Verification items for the finished model (mm, model axes). A direction names the side the tool comes from. Give positions to 0.01 mm unless a question says otherwise; leave off trailing zeros. Write each loop counter-clockwise with the first axis right and the second up, starting at its lowest first coordinate (ties: lowest second). Pieces come first, ordered by that corner, then holes.
Autodesk Inventor part; units mm, degrees
ref_plane "YZ Plane" through (0, 0, 0) normal (1, 0, 0) x (0, 1, 0)
ref_plane "XZ Plane" through (0, 0, 0) normal (0, 1, 0) x (-1, 0, 0)
ref_plane "XY Plane" through (0, 0, 0) normal (0, 0, 1) x (1, 0, 0)
sketch "Sketch1" plane through (0, 0, 0) normal (0, 0, 1) x (1, 0, 0)
  circle A0 centre (0, 0) radius 30.099
  dimension "d0" = 60.198
extrude "Extrusion1" add sketch "Sketch1" along normal blind 6.1468
sketch "Sketch2" plane through (0, 0, 0) normal (0, 0, -1) x (-1, 0, 0)
  circle A0 centre (0, 0) radius 21.3106
  dimension "d3" = 42.6212
extrude "Extrusion2" add sketch "Sketch2" along normal blind 5.08
sketch "Sketch3" plane through (0, 0, 0) normal (0, 0, -1) x (-1, 0, 0)
  circle A0 centre (0, 0) radius 21.3106
  circle A1 centre (0, 0) radius 30.099
  line L0 (0, 25.4139) -> (22.0091, -12.707) construction
  line L1 (22.0091, -12.707) -> (-22.0091, -12.707) construction
  line L2 (-22.0091, -12.707) -> (0, 25.4139) construction
  circle A2 centre (0, 25.4139) radius 1.4224
  circle A3 centre (22.0091, -12.707) radius 1.4224
  circle A4 centre (-22.0091, -12.707) radius 1.4224
  line L3 (-11.071, 20.6645) -> (5.4814, 30.221) construction
  line L4 (36.2551, -6.1245) -> (10.9127, -20.7559) construction
  dimension "d6" = 44.0182
  dimension "d7" = 2.8448
  dimension "d8" = 46.863
extrude "Extrusion3" add sketch "Sketch3" along normal blind 8.6868 contours A2 | A3 | A4
sketch "Sketch4" plane through (0, 0, 0) normal (1, 0, 0) x (0, 1, 0)
  line L0 (30.099, 6.1468) -> (-30.099, 6.1468)
  line L1 (27.2941, 6.1468) -> (19.2856, 15.3189)
  line L2 (19.2856, 15.3189) -> (19.2856, 28.4756)
  line L3 (19.2856, 28.4756) -> (0, 28.4756)
  line L4 (0, 28.4756) -> (0, 0)
  point P0 (0, 6.1468)
revolve "Revolution1" add sketch "Sketch4" angle 360 about axis through (0, 0, 28.4756) along (0, 0, -1)
sketch "Sketch5" plane through (0, 0, 28.4756) normal (0, 0, 1) x (1, 0, 0)
  circle A0 centre (0, -14.4677) radius 2.7154
  point P0 (0, 0)
extrude "Extrusion4" add sketch "Sketch5" along normal blind 16.6243
properties part number "MPG"
Item 1: Depth check by flat-ended pin: pin 1 (6 mm diameter, centred on x = 21.5, y = 19.5, fed in from -Z); pin 2 (12 mm diameter, centred on x = -3, y = -5, fed in from -Z); pin 3 (12 mm diameter, centred on y = -15, z = 13, fed in from +X). Enter the tip coordinate at first touch or a pass-through.
Answer key:
pin 1: stops at z = 0
pin 2: stops at z = -5.08
pin 3: stops at x = 22.9
Item 2: Release check for a two-part mould opening along Y. For faces 1 (the face through (-0.656, 26.676, -4.283)), 2 (the face through (0, 0, -5.08)), 3 (the face through (18.827, -4.181, 21.989)) record: released by +Y, released by -Y, zero draft, split by the parting line, or undercut.
Answer key:
face 1: undercut
face 2: zero draft
face 3: split by the parting line
Item 3: Sectioned sample at A-A on x = 0. Record the cut outline in (y, z).
Answer key:
outline: (-30.1, 0) - (-21.31, 0) - (-21.31, -5.08) - (21.31, -5.08) - (21.31, 0) - (23.99, 0) - (23.99, -8.69) - (26.84, -8.69) - (26.84, 0) - (30.1, 0) - (30.1, 6.15) - (27.29, 6.15) - (19.29, 15.32) - (19.29, 28.48) - (-11.75, 28.48) - (-11.75, 45.1) - (-17.18, 45.1) - (-17.18, 28.48) - (-19.29, 28.48) - (-19.29, 15.32) - (-27.29, 6.15) - (-30.1, 6.15) - close
Item 4: Sectioned sample at D-D on z = 23. Record the cut outline in (x, y), then the cut area to 3 significant figures.
Answer key:
outline: circle Ø38.57 at (0, 0)
area: 1,170 mm2
Item 5: Set-up check for faces 4 (the face through (-0.35, -17.16, 36.67)), 5 (the face through (-7.1, 20.5, 0)), 6 (the face through (0, -14, 45.1)): record each of +Z, -Z, +X, -X, +Y, -Y from which the full face is reachable in a straight line by a thin tool's end or side.
Answer key:
face 4: +Z
face 5: -Z
face 6: +Z, +X, -X, +Y, -Y
Item 6: Sectioned sample at B-B on y = 0. Record the cut outline in (x, z).
Answer key:
outline: (-30.1, 0) - (-21.31, 0) - (-21.31, -5.08) - (21.31, -5.08) - (21.31, 0) - (30.1, 0) - (30.1, 6.15) - (27.29, 6.15) - (19.29, 15.32) - (19.29, 28.48) - (-19.29, 28.48) - (-19.29, 15.32) - (-27.29, 6.15) - (-30.1, 6.15) - close
Item 7: Sectioned sample at C-C on z = -4. Record the cut outline in (x, y), then the cut area to 3 significant figures.
Answer key:
outline: circle Ø2.84 at (-22.01, -12.71); circle Ø42.62 at (0, 0); circle Ø2.84 at (0, 25.41); circle Ø2.84 at (22.01, -12.71)
area: 1,450 mm2
Item 8: Scan lines: line 1 along Z through (x, y) = (-5.5, -9.5); line 2 along Y through (x, z) = (22, -3); line 3 along Z through (x, y) = (-12.5, -20). Record each from-to range of solid material in increasing order.
Answer key:
line 1: z = -5.08 to 28.48
line 2: y = -14.13 to -11.28
line 3: z = 0 to 10.39
